Design review of the part built by this model. Coordinates are the model's own, in mm. Face numbers are marked on the shaded views. A direction names the side the tool comes from. Give positions to 0.01 mm unless a question says otherwise; leave off trailing zeros. Write each loop counter-clockwise with the first axis right and the second up, starting at its lowest first coordinate (ties: lowest second). Pieces come first, ordered by that corner, then holes. Notation, with made-up numbers: (-37, 84.5) -> (6, 84.5) arc R19 ccw to (6, 111.5) -> close; hole circle Ø2 at (1, -32). An arc over 180 degrees is marked (long way). Answer as a JSON object with one key per item and string values.
```python
from build123d import *

# Parameters (mm, degrees)
F1_DEPTH = 101.6
F3_D     = 6.35


with BuildPart() as f1:
    # F0 (on Front) → F1 (new body)
    with BuildSketch(Plane.XZ):
        Polygon((-9.525, 50.8), (-12.7, 50.8), (-12.7, 0), (0, 0), (0, 3.175), (-9.525, 3.175), align=None)
    extrude(amount=F1_DEPTH)

    # F3 (through all)
    with Locations(Plane(origin=(-12.7, 0, 0), x_dir=(0, -1, 0), z_dir=(-1, 0, 0))):
        with Locations((88.9, 38.1), (88.9, 12.7)):
            Hole(F3_D / 2)

    # F4: F1 across plane


with BuildPart() as f1_1:
    add(f1.part)
    add(f1.part.mirror(Plane.XZ))


solid = f1_1.part
```
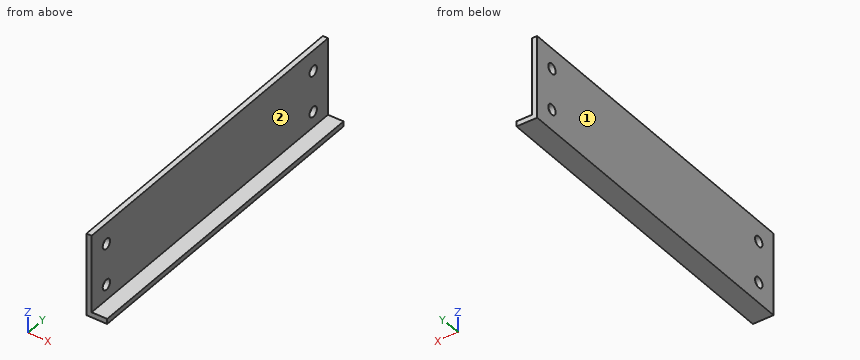
(1) We need section D-D, the plane x = -5. State the section outline as (y, z) points (3 decimals), then the cut area to 3 significant figures.
Here are the results:
{"outline": "(-101.6, 0) -> (101.6, 0) -> (101.6, 3.175) -> (-101.6, 3.175) -> close", "area": "645 mm²"}
(2) We need section C-C, the plane y = -30. State the section outline as (x, z) points (3 decimals), then the cut area to 3 significant figures.
Here are the results:
{"outline": "(-12.7, 0) -> (0, 0) -> (0, 3.175) -> (-9.525, 3.175) -> (-9.525, 50.8) -> (-12.7, 50.8) -> close", "area": "192 mm²"}
(3) We need section B-B, the plane z = 12.7. State the section outline as (x, y) points (3 decimals).
Here are the results:
{"outline": "(-12.7, -101.6) -> (-9.525, -101.6) -> (-9.525, -92.075) -> (-12.7, -92.075) -> close; (-12.7, -85.725) -> (-9.525, -85.725) -> (-9.525, 85.725) -> (-12.7, 85.725) -> close; (-12.7, 92.075) -> (-9.525, 92.075) -> (-9.525, 101.6) -> (-12.7, 101.6) -> close"}
(4) We need section A-A, the plane y = 88.9. State the section outline as (x, z) points (3 decimals), then the cut area to 3 significant figures.
Here are the results:
{"outline": "(-12.7, 0) -> (0, 0) -> (0, 3.175) -> (-9.525, 3.175) -> (-9.525, 9.525) -> (-12.7, 9.525) -> close; (-12.7, 15.875) -> (-9.525, 15.875) -> (-9.525, 34.925) -> (-12.7, 34.925) -> close; (-12.7, 41.275) -> (-9.525, 41.275) -> (-9.525, 50.8) -> (-12.7, 50.8) -> close", "area": "151 mm²"}
(5) For line 1 along Z through (x, y) = (-11.4, -88.9) (3 decimals); line 2 along X through (y, z) = (53, 21) (3 decimals); line 3 along Z through (x, y) = (-1.5, 68.5) (3 decimals), list the stretches that pass through material, from the lowest coordinate up.
Here are the results:
{"line 1": "z = 0 to 9.525, 15.875 to 34.925, 41.275 to 50.8", "line 2": "x = -12.7 to -9.525", "line 3": "z = 0 to 3.175"}
(6) Clearance check with flat-ended pins moving along their axes: pin 1 (5 mm diameter, centred on y = 18.5, z = 10.5, fed in from +X) (3 decimals); pin 2 (5 mm diameter, centred on x = -2.5, y = 71, fed in from +Z) (3 decimals); pin 3 (4 mm diameter, centred on x = -4, y = 64.5, fed in from -Z). State where each tip first meets the part, or that it passes through.
Here are the results:
{"pin 1": "stops at x = -9.525", "pin 2": "stops at z = 3.175", "pin 3": "stops at z = 0"}
(7) For the marked faces 1 and 2, list the 3-axis set-ups (+Z, -Z, +X, -X, +Y, -Y) from which the entire face can be reached by the end or side of a thin tool; tool diameter is ignored.
Here are the results:
{"face 1": "+Z, -Z, -X, +Y, -Y", "face 2": "+Z, +X, +Y, -Y"}
